Verification items for the finished model (mm, model axes). Face numbers are marked on the shaded views. A direction names the side the tool comes from. Give positions to 0.01 mm unless a question says otherwise; leave off trailing zeros. Write each loop counter-clockwise with the first axis right and the second up, starting at its lowest first coordinate (ties: lowest second). Pieces come first, ordered by that corner, then holes. Notation, with made-up numbers: (14, 19) -> (35, 19) arc R33 ccw to (35, 55) -> close; hole circle Ø10 at (26, -34). An arc over 180 degrees is marked (long way). Answer as CSV lines item,"result". Start each with the question number.
1) Sectioned sample at C-C on x = 0. Record the cut outline in (y, z).
2) Sectioned sample at B-B on y = -7.5. Record the cut outline in (x, z), and give its area (3 significant figures).
3) Material ranges on L1, parallel to X at y = -7, z = -4.75; L2, parallel to X at y = 7.75, z = -4.5; L3, parallel to Y at x = 5.5, z = -0.5, recorded low to high.
4) Mould release check, pull along X, two halves, no side actions. Record for the marked faces 1, 2, 3 and 4: released by +X, released by -X, zero draft, split by the parting line, or undercut.
5) Sectioned sample at D-D on x = -8. Record the cut outline in (y, z).
6) Tool access check on the marked faces 5, 6 and 7. Record the directions out of +Z, -Z, +X, -X, +Y, -Y that give a thin tool (end or side, any length) a straight path to the whole face; none if there is none.
7) Gauge pin test, flat ends, axial feed: pin 1 Ø7.5 at (x, y) = (0, 0) entering from -Z; pin 2 Ø8 at (x, y) = (4, 3) entering from +Z; pin 3 Ø0.8 at (x, z) = (-8.5, -3.5) entering from +Y. Record the tip position at first contact, or that the pin passes through.
8) Sectioned sample at A-A on x = 8.25. Record the cut outline in (y, z).
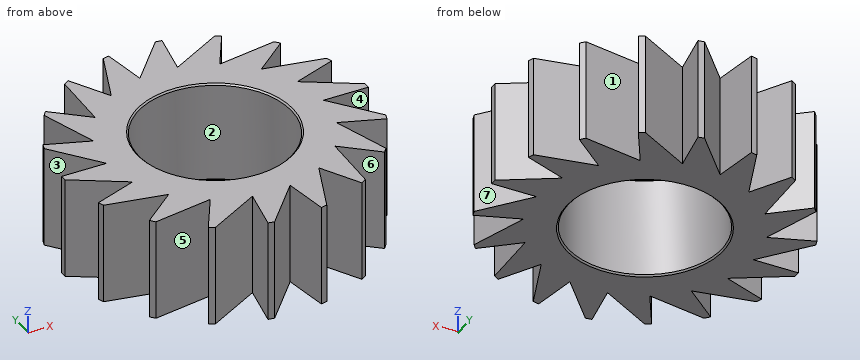
```python
from build123d import *

# Parameters (mm, degrees)
SKETCH1_R               = 6.731
SKETCH1_R_2             = 4.7625
BOSS_EXTRUDE1_DEPTH     = 6.35
BOSS_EXTRUDE2_DEPTH     = 6.35
CIRPATTERN1_COUNT       = 18
CHAMFER1_SIZE           = 0.09525
SKETCH3_R               = 314.325
SKETCH3_R_2             = 9.525
CUT_EXTRUDE_THIN1_DEPTH = 16.60964661


with BuildPart() as part:
    # Sketch1 → Boss-Extrude1 (new body)
    with BuildSketch(Plane.XY):
        Circle(SKETCH1_R)
        Circle(SKETCH1_R_2, mode=Mode.SUBTRACT)
    extrude(amount=-BOSS_EXTRUDE1_DEPTH)

    # Sketch2 → Boss-Extrude2 (add)
    with BuildSketch(Plane.XY):
        with BuildLine():
            Line((-1.168825884, 6.628740986), (1.764265485, 10.005646771))
            Line((1.764265485, 10.005646771), (1.168825884, 6.628740986))
            ThreePointArc((1.168825884, 6.628740986), (0, 6.731), (-1.168825884, 6.628740986))
        make_face()
    boss_extrude2 = extrude(amount=-BOSS_EXTRUDE2_DEPTH)

    # CirPattern1: Boss-Extrude2 ×18 about axis
    cirpattern1_axis = Axis((0, 0, 0), (0, 0, 1))
    for i in range(1, CIRPATTERN1_COUNT):
        add(boss_extrude2.rotate(cirpattern1_axis, i * 360 / CIRPATTERN1_COUNT))

    # Chamfer1
    chamfer1_edges = [part.edges().sort_by_distance(p)[0] for p in [
        (-4.7625, 0, -6.35),
        (-4.7625, 0, 0),
    ]]
    chamfer(chamfer1_edges, length=CHAMFER1_SIZE)

    # Sketch3 → Cut-Extrude-Thin1 (cut, through all)
    with BuildSketch(Plane.XY):
        Circle(SKETCH3_R)
        Circle(SKETCH3_R_2, mode=Mode.SUBTRACT)
    extrude(amount=-CUT_EXTRUDE_THIN1_DEPTH, mode=Mode.SUBTRACT)


solid = part.part
```
Ans:
1,outline,"(-7.97, -6.35) -> (-4.86, -6.35) -> (-4.76, -6.25) -> (-4.76, -0.1) -> (-4.86, 0) -> (-7.97, 0) -> close; (4.76, -6.25) -> (4.86, -6.35) -> (7.97, -6.35) -> (7.97, 0) -> (4.86, 0) -> (4.76, -0.1) -> close"
2,outline,"(-4.33, -6.35) -> (-2.74, -6.35) -> (-2.74, 0) -> (-4.33, 0) -> close; (-1.32, -6.35) -> (0.41, -6.35) -> (0.41, 0) -> (-1.32, 0) -> close; (1.32, -6.35) -> (2.72, -6.35) -> (2.72, 0) -> (1.32, 0) -> close; (4.33, -6.35) -> (5.1, -6.35) -> (5.1, 0) -> (4.33, 0) -> close"
2,area,"34.9 mm²"
3,L1,"x = -4.04 to -1.84, -1.23 to 0.85, 1.23 to 2.92, 4.04 to 5.11"
3,L2,"x = -5.1 to -4.47, -2.63 to -1.37, -0.19 to 1.37, 3.19 to 4.47"
3,L3,"y = -4.62 to 4.26, 4.62 to 6.17"
4,face 1,"undercut"
4,face 2,"undercut"
4,face 3,"released by -X"
4,face 4,"zero draft"
5,outline,"(-3.78, -6.35) -> (-2.91, -6.35) -> (-2.91, 0) -> (-3.78, 0) -> close; (-1.3, -6.35) -> (0, -6.35) -> (0, 0) -> (-1.3, 0) -> close; (1.57, -6.35) -> (2.91, -6.35) -> (2.91, 0) -> (1.57, 0) -> close"
6,face 5,"+Z, -Z"
6,face 6,"+Z, -Z, -Y"
6,face 7,"+Z, -Z, +X"
7,pin 1,"passes through"
7,pin 2,"stops at z = 0"
7,pin 3,"stops at y = 3.24"
8,outline,"(-3, -6.35) -> (-1.87, -6.35) -> (-1.87, 0) -> (-3, 0) -> close; (0, -6.35) -> (1.15, -6.35) -> (1.15, 0) -> (0, 0) -> close; (3, -6.35) -> (3.73, -6.35) -> (3.73, 0) -> (3, 0) -> close"
